Verification items for the finished model (mm, model axes). Give positions to 0.01 mm unless a question says otherwise; leave off trailing zeros. Order: outer loops, then holes, each group sorted by start corner. A loop starts at its lowest first (then second) coordinate and runs counter-clockwise, first axis right, second up. Notation, with made-up numbers: (-26.75, 75) - (-7.75, 75) arc R17 ccw to (-7.75, 91) - close; hole circle Ø7 at (13, -19). An arc over 180 degrees is marked (long way). Answer as a JSON object with one key per item and string values.
```python
from build123d import *

# Parameters (mm, degrees)
F0_W          = 380
F0_H          = 375
F0_R          = 75
F1_DEPTH      = 5
F1_DEPTH_BACK = 5


with BuildPart() as f1:
    # F0 (on Top) → F1 (new body, two sides)
    with BuildSketch(Plane.XY) as f1_sk:
        Rectangle(F0_W, F0_H)
        Circle(F0_R, mode=Mode.SUBTRACT)
    extrude(amount=F1_DEPTH)
    extrude(f1_sk.sketch, amount=-F1_DEPTH_BACK)


solid = f1.part
```
(1) Section check A-A (x = 0). Record the cut outline in (y, z), then the cut area to 3 significant figures.
Computed values:
{"outline": "(-187.5, -5) - (-75, -5) - (-75, 5) - (-187.5, 5) - close; (75, -5) - (187.5, -5) - (187.5, 5) - (75, 5) - close", "area": "2,250 mm²"}
(2) Section check C-C (z = 3.25). Record the cut outline in (x, y), then the cut area to 3 significant figures.
Computed values:
{"outline": "(-190, -187.5) - (190, -187.5) - (190, 187.5) - (-190, 187.5) - close; hole circle Ø150 at (0, 0)", "area": "125,000 mm²"}
(3) Section check B-B (y = 0). Record the cut outline in (x, z).
Computed values:
{"outline": "(-190, -5) - (-75, -5) - (-75, 5) - (-190, 5) - close; (75, -5) - (190, -5) - (190, 5) - (75, 5) - close"}
(4) Material ranges on line 1 along Y through (x, z) = (0, -3); line 2 along Y through (x, z) = (-68, 4.75); line 3 along X through (y, z) = (30, 0.5), recorded low to high. Write a range as [from, to].
Computed values:
{"line 1": "y = [-187.5, -75], [75, 187.5]", "line 2": "y = [-187.5, -31.64], [31.64, 187.5]", "line 3": "x = [-190, -68.74], [68.74, 190]"}
(5) Release check for a two-part mould opening along Y. For faces 1 (the flat face through (-190, -3, 0)), 2 (the cylindrical face through (-9.764, 74.362, -0.07)), 3 (the flat face through (-3, -187.5, 0)), 4 (the flat face through (-3, 187.5, 0)) record: pulls with the +Y half, pulls with the -Y half, needs draft (parallel to the pull), parting line crosses it, or undercut.
Computed values:
{"face 1": "needs draft", "face 2": "undercut", "face 3": "pulls with the -Y half", "face 4": "pulls with the +Y half"}
